Source: CAD feature listing. Evaluate the final solid. Frame: model axes, mm. A direction names the side the tool comes from. Give positions to 0.01 mm unless a question says otherwise; leave off trailing zeros. Write each loop counter-clockwise with the first axis right and the second up, starting at its lowest first coordinate (ties: lowest second). Pieces come first, ordered by that corner, then holes. Notation, with made-up numbers: M 36.5,-19.5 L 56.5,-19.5 A9 ccw 56.5,-11.5 Z; hole C -37,39 d8. An arc over 180 degrees is marked long. Return JSON: item names as keys, results as strings.
```python
from build123d import *

# Parameters (mm, degrees)
BOSS_EXTRUDE1_DEPTH = 710
SKETCH2_R           = 4.5
CUT_EXTRUDE1_DEPTH  = 10
CUT_EXTRUDE2_DEPTH  = 10


with BuildPart() as part:
    # Sketch1 → Boss-Extrude1 (new body)
    with BuildSketch(Plane.XY):
        Polygon((-9.285714286, 23.80952381), (-9.285714286, -26.19047619), (15.714285714, -26.19047619), (15.714285714, -23.69047619), (-6.785714286, -23.69047619), (-6.785714286, 23.80952381), align=None)
    extrude(amount=BOSS_EXTRUDE1_DEPTH)

    # Sketch2 → Cut-Extrude1 (cut)
    with BuildSketch(Plane(origin=(-6.785714286, 0, 0), x_dir=(0, 0, -1), z_dir=(1, 0, 0))):
        with Locations(Location((-649.198051525, 6.719410966, 0), (0, 0, 90))):
            Circle(SKETCH2_R)
        with Locations(Location((-612.198051525, 6.716309021, 0), (0, 0, 90))):
            Circle(SKETCH2_R)
        with Locations(Location((-575.198051525, 6.713207076, 0), (0, 0, 90))):
            Circle(SKETCH2_R)
        with Locations(Location((-242.198051785, 6.685289571, 0), (0, 0, 90))):
            Circle(SKETCH2_R)
        with Locations(Location((-279.198051785, 6.688391516, 0), (0, 0, 90))):
            Circle(SKETCH2_R)
        with Locations(Location((-538.198051525, 6.710105131, 0), (0, 0, 90))):
            Circle(SKETCH2_R)
        with Locations(Location((-501.198051525, 6.707003186, 0), (0, 0, 90))):
            Circle(SKETCH2_R)
        with Locations(Location((-464.198051525, 6.703901241, 0), (0, 0, 90))):
            Circle(SKETCH2_R)
        with Locations(Location((-427.198051525, 6.700799296, 0), (0, 0, 90))):
            Circle(SKETCH2_R)
        with Locations(Location((-390.198051525, 6.697697351, 0), (0, 0, 90))):
            Circle(SKETCH2_R)
        with Locations(Location((-353.198051655, 6.694595406, 0), (0, 0, 90))):
            Circle(SKETCH2_R)
        with Locations(Location((-316.198051785, 6.691493461, 0), (0, 0, 90))):
            Circle(SKETCH2_R)
        with Locations(Location((-686.198051395, 6.722512911, 0), (0, 0, 90))):
            Circle(SKETCH2_R)
        with Locations(Location((-24.198051395, 6.667013246, 0), (0, 0, 90))):
            Circle(SKETCH2_R)
        with Locations(Location((-57.198052435, 6.669779846, 0), (0, 0, 90))):
            Circle(SKETCH2_R)
        with Locations(Location((-205.198051915, 6.682187626, 0), (0, 0, 90))):
            Circle(SKETCH2_R)
        with Locations(Location((-168.198052045, 6.679085681, 0), (0, 0, 90))):
            Circle(SKETCH2_R)
        with Locations(Location((-131.198052175, 6.675983736, 0), (0, 0, 90))):
            Circle(SKETCH2_R)
        with Locations(Location((-94.198052305, 6.672881791, 0), (0, 0, 90))):
            Circle(SKETCH2_R)
    extrude(amount=-CUT_EXTRUDE1_DEPTH, mode=Mode.SUBTRACT)

    # Sketch3 → Cut-Extrude2 (cut)
    with BuildSketch(Plane(origin=(0, -23.69047619, 0), x_dir=(1, 0, 0), z_dir=(0, 1, 0))):
        with BuildLine():
            Line((0.964285714, -220.615260366), (0.964285714, -201.615260366))
            ThreePointArc((0.964285714, -201.615260366), (4.464285714, -198.163676075), (7.964285714, -201.615260366))
            Line((7.964285714, -201.615260366), (7.964285714, -220.615260366))
            ThreePointArc((7.964285714, -220.615260366), (4.464285714, -224.19719897), (0.964285714, -220.615260366))
        make_face()
        with BuildLine():
            Line((0.963115287, -134.265755564), (0.964027858, -115.265755586))
            ThreePointArc((0.964027858, -115.265755586), (4.465316374, -111.767044577), (7.964027383, -115.268333093))
            Line((7.964027383, -115.268333093), (7.965046039, -134.268333066))
            ThreePointArc((7.965046039, -134.268333066), (4.462738275, -137.913718588), (0.963115287, -134.265755564))
        make_face()
        with BuildLine():
            Line((1.116372812, -42.705779315), (1.116372812, -24.705779315))
            ThreePointArc((1.116372812, -24.705779315), (4.616372812, -21.205779315), (8.116372812, -24.705779315))
            Line((8.116372812, -24.705779315), (8.116372812, -42.705779315))
            ThreePointArc((8.116372812, -42.705779315), (4.616372812, -46.205779315), (1.116372812, -42.705779315))
        make_face()
        with BuildLine():
            Line((0.944319512, -305.018833037), (0.944319512, -286.018833037))
            ThreePointArc((0.944319512, -286.018833037), (4.444319512, -282.567248747), (7.944319512, -286.018833037))
            Line((7.944319512, -286.018833037), (7.944319512, -305.018833037))
            ThreePointArc((7.944319512, -305.018833037), (4.444319512, -308.600771642), (0.944319512, -305.018833037))
        make_face()
        with BuildLine():
            Line((0.942476542, -377.078536786), (0.942476542, -358.078536786))
            ThreePointArc((0.942476542, -358.078536786), (4.442476542, -354.626952496), (7.942476542, -358.078536786))
            Line((7.942476542, -358.078536786), (7.942476542, -377.078536786))
            ThreePointArc((7.942476542, -377.078536786), (4.442476542, -380.660475391), (0.942476542, -377.078536786))
        make_face()
        with BuildLine():
            Line((0.937060946, -461.70401329), (0.937060946, -442.70401329))
            ThreePointArc((0.937060946, -442.70401329), (4.437060946, -439.252429), (7.937060946, -442.70401329))
            Line((7.937060946, -442.70401329), (7.937060946, -461.70401329))
            ThreePointArc((7.937060946, -461.70401329), (4.437060946, -465.285951895), (0.937060946, -461.70401329))
        make_face()
        with BuildLine():
            Line((0.982865657, -549.330591868), (0.982865657, -530.330591868))
            ThreePointArc((0.982865657, -530.330591868), (4.482865657, -526.879007577), (7.982865657, -530.330591868))
            Line((7.982865657, -530.330591868), (7.982865657, -549.330591868))
            ThreePointArc((7.982865657, -549.330591868), (4.482865657, -552.912530473), (0.982865657, -549.330591868))
        make_face()
        with BuildLine():
            Line((0.930766494, -629.221929405), (0.930766494, -610.221929405))
            ThreePointArc((0.930766494, -610.221929405), (4.430766494, -606.770345115), (7.930766494, -610.221929405))
            Line((7.930766494, -610.221929405), (7.930766494, -629.221929405))
            ThreePointArc((7.930766494, -629.221929405), (4.430766494, -632.80386801), (0.930766494, -629.221929405))
        make_face()
        with BuildLine():
            Line((0.92534668, -692.195222709), (0.92534668, -673.195222709))
            ThreePointArc((0.92534668, -673.195222709), (4.42534668, -669.743638419), (7.92534668, -673.195222709))
            Line((7.92534668, -673.195222709), (7.92534668, -692.195222709))
            ThreePointArc((7.92534668, -692.195222709), (4.42534668, -695.777161314), (0.92534668, -692.195222709))
        make_face()
    extrude(amount=-CUT_EXTRUDE2_DEPTH, mode=Mode.SUBTRACT)


solid = part.part
```
1) Cut plane B-B, the plane z = 486. Return the cut outline in (x, y), then the cut area to 3 significant figures.
Numbers:
{"outline": "M -9.29,-26.19 L 15.71,-26.19 L 15.71,-23.69 L -6.79,-23.69 L -6.79,23.81 L -9.29,23.81 Z", "area": "181 mm²"}
2) Line query: line 1 (X direction, y = -4, z = 306.5); line 2 (Y direction, x = 12.5, z = 247.5). Output: solid intervals per line, ascending. Write a range as [from, to].
Numbers:
{"line 1": "x = [-9.29, -6.79]", "line 2": "y = [-26.19, -23.69]"}
3) Cut plane A-A, the plane z = 365.5. Return the cut outline in (x, y).
Numbers:
{"outline": "M -9.29,-26.19 L 0.94,-26.19 L 0.94,-23.69 L -6.79,-23.69 L -6.79,23.81 L -9.29,23.81 Z; M 7.94,-26.19 L 15.71,-26.19 L 15.71,-23.69 L 7.94,-23.69 Z"}
4) Cut plane D-D, the plane y = -17. Return the cut outline in (x, z), then the cut area to 4 significant figures.
Numbers:
{"outline": "M -9.29,0 L -6.79,0 L -6.79,710 L -9.29,710 Z", "area": "1,775 mm²"}
5) Cut plane C-C, the plane x = -3. Return the cut outline in (y, z), then the cut area to 4 significant figures.
Numbers:
{"outline": "M -26.19,0 L -23.69,0 L -23.69,710 L -26.19,710 Z", "area": "1,775 mm²"}
6) Set-up query: faces 1 (the face through (-7, -7, 0)), 2 (the face through (-6.786, 0, 350)). Return all of +Z, -Z, +X, -X, +Y, -Y with unobstructed straight access to the full face (end or side cutting, diameter ignored); none if empty.
Numbers:
{"face 1": "-Z, +X, -X, +Y, -Y", "face 2": "+Z, -Z, +X, +Y"}
7) Contact query for flat-ended pins moving along their axis: pin 1 Ø7 at (y, z) = (6.71, 575.2) entering from +X; pin 2 Ø2 at (y, z) = (-1, 629.5) entering from +X; pin 3 Ø1 at (x, z) = (2.5, 514.5) entering from +Y. Output: stop coordinate, or through.
Numbers:
{"pin 1": "passes through", "pin 2": "stops at x = -6.79", "pin 3": "stops at y = -23.69"}
